from build123d import *

# Parameters (mm, degrees)
F0_W     = 106.68
F0_H     = 52.832
F0_W_2   = 99.06
F0_H_2   = 45.212
F1_DEPTH = 12.7
F2_W     = 99.06
F2_H     = 45.212
F3_DEPTH = 2.54
F4_W     = 3.81
F4_H     = 6.35
F5_DEPTH = 10.16
F6_R     = 2.54


with BuildPart() as f1:
    # F0 (on Top) → F1 (new body)
    with BuildSketch(Plane.XY):
        Rectangle(F0_W, F0_H)
        Rectangle(F0_W_2, F0_H_2, mode=Mode.SUBTRACT)
    extrude(amount=F1_DEPTH)

    # F2 (on Top) → F3 (join)
    with BuildSketch(Plane.XY):
        Rectangle(F2_W, F2_H)
    extrude(amount=F3_DEPTH)

    # F4 (on face) → F5 (cut)
    with BuildSketch(Plane.XY.offset(12.7)):
        with Locations((51.435, 19.431)):
            Rectangle(F4_W, F4_H)
        with Locations((51.435, -19.431)):
            Rectangle(F4_W, F4_H)
    extrude(amount=-F5_DEPTH, mode=Mode.SUBTRACT)

    # F6 (call 1 of 8: OpenCascade refuses the feature's edges together)
    f6_edges = [f1.edges().sort_by_distance(p)[0] for p in [
        (49.53, 16.256, 7.62),
    ]]
    fillet(f6_edges, radius=F6_R)

    # F6#2 (call 2 of 8)
    f6_2_edges = [f1.edges().sort_by_distance(p)[0] for p in [
        (53.34, 22.606, 7.62),
    ]]
    fillet(f6_2_edges, radius=F6_R)

    # F6#3 (call 3 of 8)
    f6_3_edges = [f1.edges().sort_by_distance(p)[0] for p in [
        (49.53, -16.256, 7.62),
    ]]
    fillet(f6_3_edges, radius=F6_R)

    # F6#4 (call 4 of 8)
    f6_4_edges = [f1.edges().sort_by_distance(p)[0] for p in [
        (53.34, -22.606, 7.62),
    ]]
    fillet(f6_4_edges, radius=F6_R)

    # F6#5 (call 5 of 8)
    f6_5_edges = [f1.edges().sort_by_distance(p)[0] for p in [
        (53.34, 26.416, 6.35),
    ]]
    fillet(f6_5_edges, radius=F6_R)

    # F6#6 (call 6 of 8)
    f6_6_edges = [f1.edges().sort_by_distance(p)[0] for p in [
        (53.34, -26.416, 6.35),
    ]]
    fillet(f6_6_edges, radius=F6_R)

    # F6#7 (call 7 of 8)
    f6_7_edges = [f1.edges().sort_by_distance(p)[0] for p in [
        (-53.34, -26.416, 6.35),
    ]]
    fillet(f6_7_edges, radius=F6_R)

    # F6#8 (call 8 of 8)
    f6_8_edges = [f1.edges().sort_by_distance(p)[0] for p in [
        (-53.34, 26.416, 6.35),
    ]]
    fillet(f6_8_edges, radius=F6_R)


solid = f1.part
For this review, take the finished solid that the model builds, in its own axes (mm). A direction names the side the tool comes from. Give positions to 0.01 mm unless a question says otherwise; leave off trailing zeros. Loops run counter-clockwise (first coordinate to the right, second up) from the corner with the lowest first, then second, coordinate; pieces in that order, holes last. Notation, with made-up numbers: (31, 47) -> (89, 47) arc R31 cw to (89, 84) -> close; hole circle Ø6 at (16.5, 24). An arc over 180 degrees is marked (long way). One line per question, with ' | ' between items.
1) To check wall thickness, follow probe 1 along X at (y, z) = (-9, 7.75); probe 2 along Y at (x, z) = (-41, 11.75); probe 3 along Z at (x, y) = (18, 18). State the ranges of each line that lie inside material, in increasing order.
Resolved:
probe 1: x = -53.34 to -49.53, 49.53 to 53.34 | probe 2: y = -26.42 to -22.61, 22.61 to 26.42 | probe 3: z = 0 to 2.54
2) The part is to be moulded in two halves that separate along X. For faces 4 (the cylindrical face through (50.25, 15.49, 7.55)), 5 (the flat face through (-1, -26.416, 6)), 6 (the flat face through (53.34, 0, 6)), say which applies: +X half, -X half, draft (parallel to the pull), parting line (faces both ways), or undercut.
Resolved:
face 4: undercut | face 5: draft | face 6: +X half
3) We need section D-D (y = -18). Write out the cut boundary in (x, z).
Resolved:
outline: (-53.34, 0) -> (53.34, 0) -> (53.34, 2.54) -> (-49.53, 2.54) -> (-49.53, 12.7) -> (-53.34, 12.7) -> close
4) Insertion check: pin 1 Ø1.5 at (x, y) = (-42, 2) entering from -Z; pin 2 Ø24.5 at (x, y) = (14.5, -9.5) entering from +Z. Each pin has a flat end and moves straight along its axis. Give the tip position at first contact, or say it passes through.
Resolved:
pin 1: stops at z = 0 | pin 2: stops at z = 2.54
5) We need section A-A (z = 4.5). Write out the cut boundary in (x, y), plus the area to 3 significant figures.
Resolved:
outline: (-53.34, -23.88) arc R2.54 ccw to (-50.8, -26.42) -> (50.8, -26.42) arc R2.54 ccw to (53.26, -24.51) arc R2.54 ccw to (50.8, -22.61) -> (-49.53, -22.61) -> (-49.53, 22.61) -> (50.8, 22.61) arc R2.54 ccw to (53.26, 24.51) arc R2.54 ccw to (50.8, 26.42) -> (-50.8, 26.42) arc R2.54 ccw to (-53.34, 23.88) -> close; (49.53, -13.72) arc R2.54 ccw to (52.07, -16.26) -> (53.34, -16.26) -> (53.34, 16.26) -> (52.07, 16.26) arc R2.54 ccw to (49.53, 13.72) -> close | area: 1,100 mm2
6) We need section C-C (x = 43). Write out the cut boundary in (y, z).
Resolved:
outline: (-26.42, 0) -> (26.42, 0) -> (26.42, 12.7) -> (22.61, 12.7) -> (22.61, 2.54) -> (-22.61, 2.54) -> (-22.61, 12.7) -> (-26.42, 12.7) -> close
7) We need section B-B (y = -3). Write out the cut boundary in (x, z).
Resolved:
outline: (-53.34, 0) -> (53.34, 0) -> (53.34, 12.7) -> (49.53, 12.7) -> (49.53, 2.54) -> (-49.53, 2.54) -> (-49.53, 12.7) -> (-53.34, 12.7) -> close
8) For faces 1 (the flat face through (-49.53, 0, 8)), 2 (the flat face through (0, -22.606, 8)), 3 (the flat face through (-53.34, 0, 6)), list the 3-axis set-ups (+Z, -Z, +X, -X, +Y, -Y) from which the entire face can be reached by the end or side of a thin tool; tool diameter is ignored.
Resolved:
face 1: +Z | face 2: +Z, +X | face 3: +Z, -Z, -X, +Y, -Y
